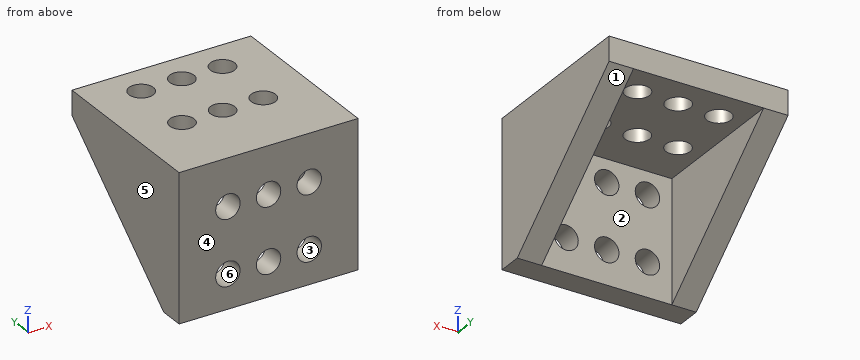
from build123d import *

# Parameters (mm, degrees)
EXTRUDE_1_DEPTH     = 22
SKETCH_2_R          = 1.5
CUT_EXTRUDE_1_DEPTH = 13
EXTRUDE_2_DEPTH     = 3
EXTRUDE_3_DEPTH     = 3
SKETCH_5_R          = 1.5
CUT_EXTRUDE_2_DEPTH = 3


with BuildPart() as part:
    # 草图1 → 凸台-拉伸1 (new body)
    with BuildSketch(Plane(origin=(0, 0, 0), x_dir=(0, 0, -1), z_dir=(1, 0, 0))):
        Polygon((0, 0), (0, 21), (3, 21), (3, 3), (18, 3), (18, 0), align=None)
    extrude(amount=EXTRUDE_1_DEPTH)

    # 草图2 → 切除-拉伸1 (cut)
    with BuildSketch(Plane(origin=(0, 3, 0), x_dir=(1, 0, 0), z_dir=(0, 1, 0))):
        with Locations(Location((11, 5.8, 0), (0, 0, 270))):
            Circle(SKETCH_2_R)
        with Locations(Location((11, 13.8, 0), (0, 0, 270))):
            Circle(SKETCH_2_R)
        with Locations(Location((16, 5.8, 0), (0, 0, 270))):
            Circle(SKETCH_2_R)
        with Locations(Location((16, 13.8, 0), (0, 0, 270))):
            Circle(SKETCH_2_R)
        with Locations(Location((6, 13.8, 0), (0, 0, 270))):
            Circle(SKETCH_2_R)
        with Locations(Location((6, 5.8, 0), (0, 0, 270))):
            Circle(SKETCH_2_R)
    extrude(amount=-CUT_EXTRUDE_1_DEPTH, mode=Mode.SUBTRACT)

    # 草图3 → 凸台-拉伸2 (add)
    with BuildSketch(Plane(origin=(22, 0, 0), x_dir=(0, 0, -1), z_dir=(1, 0, 0))):
        Polygon((3, 21), (18, 3), (3, 3), align=None)
    extrude(amount=-EXTRUDE_2_DEPTH)

    # 草图4 → 凸台-拉伸3 (add)
    with BuildSketch(Plane.ZY):
        Polygon((-18, 3), (-3, 3), (-3, 21), align=None)
    extrude(amount=-EXTRUDE_3_DEPTH)

    # 草图5 → 切除-拉伸2 (cut)
    with BuildSketch(Plane.XY):
        with Locations((11, 17)):
            Circle(SKETCH_5_R)
        with Locations((11, 9)):
            Circle(SKETCH_5_R)
        with Locations((6, 17)):
            Circle(SKETCH_5_R)
        with Locations((6, 9)):
            Circle(SKETCH_5_R)
        with Locations(Location((16, 9, 0), (0, 0, 180))):
            Circle(SKETCH_5_R)
        with Locations(Location((16, 17, 0), (0, 0, 180))):
            Circle(SKETCH_5_R)
    extrude(amount=-CUT_EXTRUDE_2_DEPTH, mode=Mode.SUBTRACT)


solid = part.part
Source: CAD feature listing. Evaluate the final solid. Frame: model axes, mm. Face numbers are marked on the shaded views. A direction names the side the tool comes from. Coordinates: 2 decimals unless noted, no trailing zeros. Loops run counter-clockwise (first coordinate to the right, second up) from the corner with the lowest first, then second, coordinate; pieces in that order, holes last. Notation, with made-up numbers: (88.5, -6) -> (133.5, -6) arc R16 ccw to (133.5, 17) -> close; hole circle Ø9 at (72.25, -30.5). An arc over 180 degrees is marked (long way). Answer in a Markdown table with one row per item. Add a question column.
Q1. Contact query for flat-ended pins moving along their axis: pin 1 Ø1.8 at (x, z) = (6, -13.8) entering from +Y; pin 2 Ø1.5 at (x, y) = (3, 17.5) entering from -Z; pin 3 Ø4.5 at (x, z) = (9, -7) entering from +Y. Output: stop coordinate, or through.
Q2. Reachability of the marked faces 1 and 2 from +Z, -Z, +X, -X, +Y, -Y: full face, straight path, thin tool, end or side. Return the list, or none.
Q3. Section D-D on z = -2.25. Return the cut outline in (x, y).
Q4. Pull-direction query (X, two-part tool) for the marked faces 3, 4, 5 and 6; classes: pulls with the +X half, pulls with the -X half, needs draft (parallel to the pull), parting line crosses it, or undercut.
Q5. Ray query, line 1 along X through (y, z) = (0.65, -5.8); line 2 along Y through (x, z) = (11, -1); line 3 along X through (y, z) = (9, -9). Return the intervals inside material, ascending.
Q6. Section A-A on z = -5.8. Return the cut outline in (x, y), and give its area (3 significant figures).
Q7. Section B-B on y = 9. Return the cut outline in (x, z).
Q8. Section C-C on x = 16. Return the cut outline in (y, z), and give its area (3 significant figures).
Computed values:
| question | item | result |
|---|---|---|
| 1 | pin 1 | passes through |
| 1 | pin 2 | stops at z = -6.54 |
| 1 | pin 3 | stops at y = 3 |
| 2 | face 1 | -Z, +X, -X, +Y |
| 2 | face 2 | -Z, +Y |
| 3 | outline | (0, 0) -> (22, 0) -> (22, 21) -> (0, 21) -> close; hole circle Ø3 at (6, 9); hole circle Ø3 at (6, 17); hole circle Ø3 at (11, 9); hole circle Ø3 at (11, 17); hole circle Ø3 at (16, 9); hole circle Ø3 at (16, 17) |
| 4 | face 3 | undercut |
| 4 | face 4 | needs draft |
| 4 | face 5 | pulls with the -X half |
| 4 | face 6 | undercut |
| 5 | line 1 | x = 0 to 4.5, 7.5 to 9.5, 12.5 to 14.5, 17.5 to 22 |
| 5 | line 2 | y = 0 to 7.5, 10.5 to 15.5, 18.5 to 21 |
| 5 | line 3 | x = 0 to 3, 19 to 22 |
| 6 | outline | (0, 0) -> (4.5, 0) -> (4.5, 3) -> (3, 3) -> (3, 17.64) -> (0, 17.64) -> close; (7.5, 0) -> (9.5, 0) -> (9.5, 3) -> (7.5, 3) -> close; (12.5, 0) -> (14.5, 0) -> (14.5, 3) -> (12.5, 3) -> close; (17.5, 0) -> (22, 0) -> (22, 17.64) -> (19, 17.64) -> (19, 3) -> (17.5, 3) -> close |
| 6 | area | 127 mm^2 |
| 7 | outline | (0, -13) -> (3, -13) -> (3, -3) -> (4.5, -3) -> (4.5, 0) -> (0, 0) -> close; (7.5, -3) -> (9.5, -3) -> (9.5, 0) -> (7.5, 0) -> close; (12.5, -3) -> (14.5, -3) -> (14.5, 0) -> (12.5, 0) -> close; (17.5, -3) -> (19, -3) -> (19, -13) -> (22, -13) -> (22, 0) -> (17.5, 0) -> close |
| 8 | outline | (0, -18) -> (3, -18) -> (3, -15.3) -> (0, -15.3) -> close; (0, -12.3) -> (3, -12.3) -> (3, -7.3) -> (0, -7.3) -> close; (0, -4.3) -> (3, -4.3) -> (3, -3) -> (7.5, -3) -> (7.5, 0) -> (0, 0) -> close; (10.5, -3) -> (15.5, -3) -> (15.5, 0) -> (10.5, 0) -> close; (18.5, -3) -> (21, -3) -> (21, 0) -> (18.5, 0) -> close |
| 8 | area | 72.0 mm^2 |
